Check sheet for the modelled part. Datum: model origin and axes. Units: mm. Face numbers are marked on the shaded views. Round coordinates to 2 decimals unless told otherwise and drop trailing zeros. Order: outer loops, then holes, each group sorted by start corner. A loop starts at its lowest first (then second) coordinate and runs counter-clockwise, first axis right, second up. Notation, with made-up numbers: (29.25, 86) -> (77.25, 86) arc R13 cw to (77.25, 90) -> close; hole circle Ø1 at (87, 29). An arc over 180 degrees is marked (long way). Use CSV: the item, a comma, the result in double quotes.
```python
from build123d import *

# Parameters (mm, degrees)
SKETCH2_W               = 20
SKETCH2_H               = 8
SKETCH2_W_2             = 16
SKETCH2_H_2             = 4
BOSS_EXTRUDE2_DEPTH     = 65
CUT_EXTRUDE2_DEPTH      = 2
SKETCH5_W               = 7.5
SKETCH5_H               = 8
BOSS_EXTRUDE3_DEPTH     = 3
SKETCH6_W               = 20
SKETCH6_H               = 8
BOSS_EXTRUDE4_DEPTH     = 10
SKETCH7_R               = 2.5
CUT_EXTRUDE3_DEPTH      = 1
CUT_EXTRUDE3_DEPTH_BACK = 9


with BuildPart() as part:
    # Sketch2 → Boss-Extrude2 (new body)
    with BuildSketch(Plane(origin=(0, 0, 0), x_dir=(1, 0, 0), z_dir=(0, 1, 0))):
        Rectangle(SKETCH2_W, SKETCH2_H)
        Rectangle(SKETCH2_W_2, SKETCH2_H_2, mode=Mode.SUBTRACT)
    extrude(amount=BOSS_EXTRUDE2_DEPTH)

    # Sketch4 → Cut-Extrude2 (cut)
    with BuildSketch(Plane(origin=(0, 0, -4), x_dir=(-1, 0, 0), z_dir=(0, 0, -1))):
        Polygon((8, 60), (-8, 60), (-8, 57.5), (-2.5, 57.5), (-2.5, 0), (2.5, 0), (2.5, 57.5), (8, 57.5), align=None)
    extrude(amount=-CUT_EXTRUDE2_DEPTH, mode=Mode.SUBTRACT)

    # Sketch5 → Boss-Extrude3 (add)
    with BuildSketch(Plane.XZ):
        with Locations((-6.25, 0)):
            Rectangle(SKETCH5_W, SKETCH5_H)
        with Locations((6.25, 0)):
            Rectangle(SKETCH5_W, SKETCH5_H)
    extrude(amount=BOSS_EXTRUDE3_DEPTH)

    # Sketch6 → Boss-Extrude4 (add)
    with BuildSketch(Plane(origin=(0, 65, 0), x_dir=(1, 0, 0), z_dir=(0, 1, 0))):
        Rectangle(SKETCH6_W, SKETCH6_H)
    extrude(amount=BOSS_EXTRUDE4_DEPTH)

    # Sketch7 → Cut-Extrude3 (cut, two sides)
    with BuildSketch(Plane(origin=(0, 0, -4), x_dir=(-1, 0, 0), z_dir=(0, 0, -1))) as cut_extrude3_sk:
        with Locations((0, 70)):
            Circle(SKETCH7_R)
    extrude(amount=CUT_EXTRUDE3_DEPTH, mode=Mode.SUBTRACT)
    extrude(cut_extrude3_sk.sketch, amount=-CUT_EXTRUDE3_DEPTH_BACK, mode=Mode.SUBTRACT)


solid = part.part
```
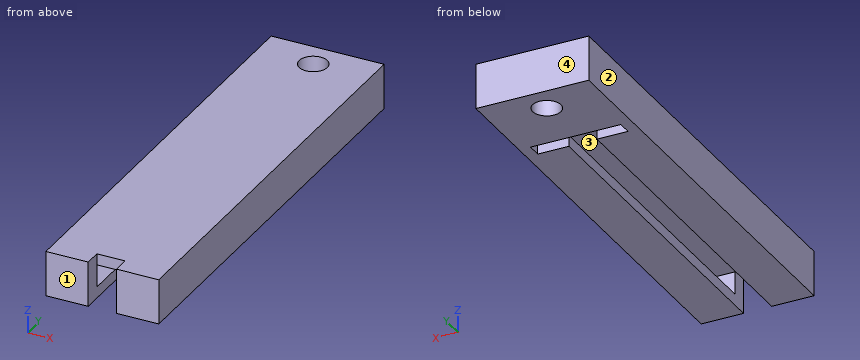
Q1. Go/stop test with flat-tipped pins: pin 1 (2 mm diameter, centred on x = 0, z = -0.5, fed in from -Y); pin 2 (0.6 mm diameter, centred on x = 1, z = -3, fed in from -Y). Record where each tip stops, or that it passes through.
Result sheet:
pin 1,"stops at y = 65"
pin 2,"stops at y = 60"
Q2. Sectioned sample at B-B, the plane z = -0.5. Enter the section's corners in (x, y), then the cut area to 3 significant figures.
Result sheet:
outline,"(-10, -3) -> (-2.5, -3) -> (-2.5, 0) -> (-8, 0) -> (-8, 65) -> (8, 65) -> (8, 0) -> (2.5, 0) -> (2.5, -3) -> (10, -3) -> (10, 75) -> (-10, 75) -> close; hole circle Ø5 at (0, 70)"
area,"485 mm^2"
Q3. Sectioned sample at C-C, the plane x = 0. Enter the section's corners in (y, z), then the cut area to 3 significant figures.
Result sheet:
outline,"(0, 2) -> (65, 2) -> (65, -2) -> (60, -2) -> (60, -4) -> (67.5, -4) -> (67.5, 4) -> (0, 4) -> close; (72.5, -4) -> (75, -4) -> (75, 4) -> (72.5, 4) -> close"
area,"180 mm^2"
Q4. Scan lines: L1, parallel to Y at x = -5, z = -3.25; L2, parallel to X at y = 19, z = -0.5; L3, parallel to Z at x = 5.5, y = 63. Record each from-to range of solid material in increasing order.
Result sheet:
L1,"y = -3 to 57.5, 60 to 75"
L2,"x = -10 to -8, 8 to 10"
L3,"z = -4 to -2, 2 to 4"
Q5. Mould release check, pull along Y, two halves, no side actions. Record for the marked faces 1, 2, 3 and 4: pulls with the +Y half, pulls with the -Y half, needs draft (parallel to the pull), parting line crosses it, or undercut.
Result sheet:
face 1,"pulls with the -Y half"
face 2,"needs draft"
face 3,"undercut"
face 4,"pulls with the +Y half"
Q6. Sectioned sample at A-A, the plane y = 70. Enter the section's corners in (x, z), then the cut area to 3 significant figures.
Result sheet:
outline,"(-10, -4) -> (-2.5, -4) -> (-2.5, 4) -> (-10, 4) -> close; (2.5, -4) -> (10, -4) -> (10, 4) -> (2.5, 4) -> close"
area,"120 mm^2"
Q7. Sectioned sample at D-D, the plane y = 26.5. Enter the section's corners in (x, z).
Result sheet:
outline,"(-10, -4) -> (-2.5, -4) -> (-2.5, -2) -> (-8, -2) -> (-8, 2) -> (8, 2) -> (8, -2) -> (2.5, -2) -> (2.5, -4) -> (10, -4) -> (10, 4) -> (-10, 4) -> close"
